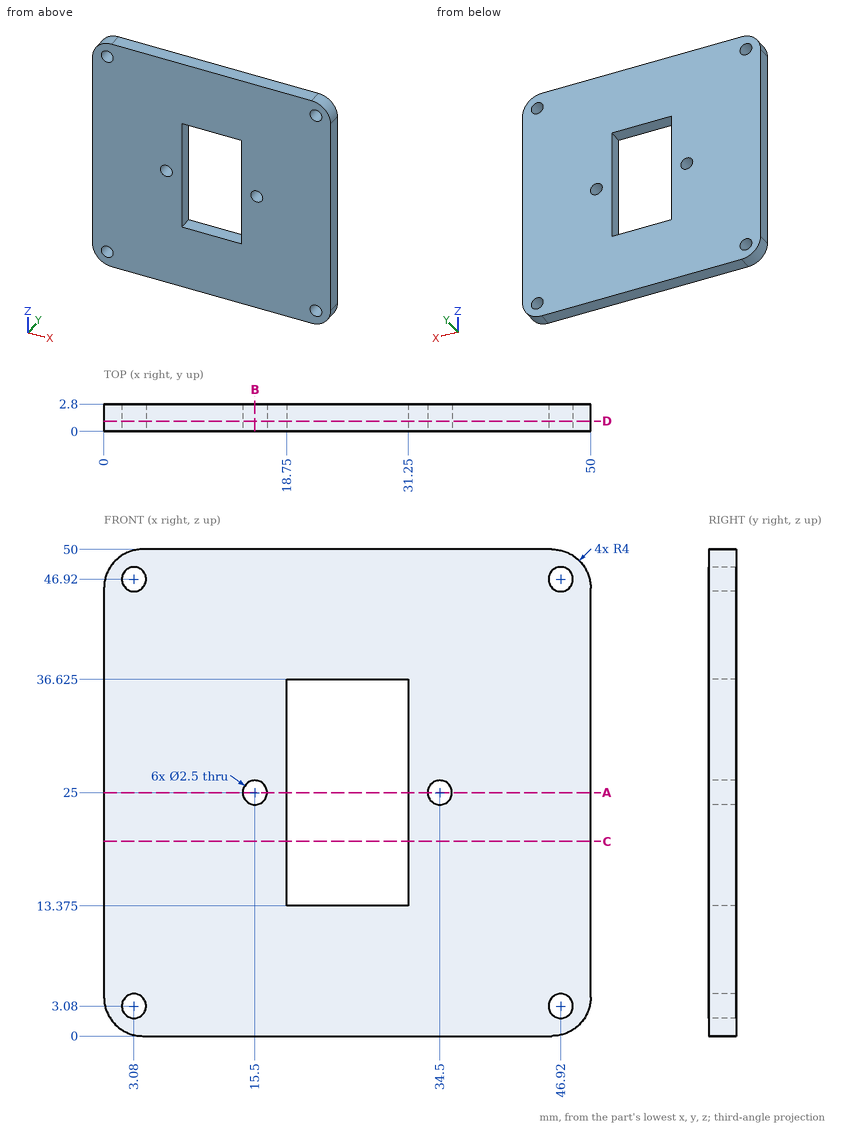
Print and shaded views of the part. All mm, measured from the part's lowest x, y and z. Round coordinates to 2 decimals unless told otherwise and drop trailing zeros. Write each loop counter-clockwise with the first axis right and the second up, starting at its lowest first coordinate (ties: lowest second). Pieces come first, ordered by that corner, then holes.
(1) Probe line 1 along X through (y, z) = (1, 18.5); line 2 along Z through (x, y) = (29.5, 1.75) (1 decimal); line 3 along X through (y, z) = (0.65, 25). List the from-to ranges inside material, lowest first.
(2) Slice it at B-B, the plane x = 15.5. Write the cut outline in (y, z).
(3) Slice it at D-D, the plane y = 1.05. Count the separate pieces of the cut face and the enclosed holes in it, and give its area (3 significant figures).
(4) Slice it at A-A, the plane z = 25. Write the cut outline in (x, y).
(5) Slice it at C-C, the plane z = 20. Write the cut outline in (x, y).
From the geometry:
1. line 1: x = 0 to 18.75, 31.25 to 50
1. line 2: z = 0 to 13.4, 36.6 to 50
1. line 3: x = 0 to 14.25, 16.75 to 18.75, 31.25 to 33.25, 35.75 to 50
2. outline: (0, 0) - (2.8, 0) - (2.8, 23.75) - (0, 23.75) - close; (0, 26.25) - (2.8, 26.25) - (2.8, 50) - (0, 50) - close
3. separate pieces: 1
3. enclosed holes: 7
3. area: 2,170 mm2
4. outline: (0, 0) - (14.25, 0) - (14.25, 2.8) - (0, 2.8) - close; (16.75, 0) - (18.75, 0) - (18.75, 2.8) - (16.75, 2.8) - close; (31.25, 0) - (33.25, 0) - (33.25, 2.8) - (31.25, 2.8) - close; (35.75, 0) - (50, 0) - (50, 2.8) - (35.75, 2.8) - close
5. outline: (0, 0) - (18.75, 0) - (18.75, 2.8) - (0, 2.8) - close; (31.25, 0) - (50, 0) - (50, 2.8) - (31.25, 2.8) - close
